```python
from build123d import *

# Parameters (mm, degrees)
SKETCH1_W                        = 99.549072562
SKETCH1_H                        = 80.386282086
EXTRUDE2_DEPTH                   = 19.05
SKETCH2_R                        = 22.2631
EXTRUDE3_DEPTH                   = 20.05
F_12_24_TAPPED_HOLE1_D           = 5.4864
F_12_24_TAPPED_HOLE1_CSINK_D     = 6.7564
F_12_24_TAPPED_HOLE1_CSINK_ANGLE = 90


with BuildPart() as part:
    # Sketch1 → Extrude2 (new body)
    with BuildSketch(Plane.XY):
        Rectangle(SKETCH1_W, SKETCH1_H)
    extrude(amount=EXTRUDE2_DEPTH)

    # Sketch2 → Extrude3 (cut, through all)
    with BuildSketch(Plane.XY.offset(19.05)):
        Circle(SKETCH2_R)
    extrude(amount=-EXTRUDE3_DEPTH, mode=Mode.SUBTRACT)

    # #12-24 Tapped Hole1 (through all)
    with Locations(Plane(origin=(49.774536281, 32.984966891, 9.857222688), x_dir=(0, 0, 1), z_dir=(1, 0, 0))):
        with Locations((0, 0), (0.189841536, 64.64104303)):
            CounterSinkHole(F_12_24_TAPPED_HOLE1_D / 2, F_12_24_TAPPED_HOLE1_CSINK_D / 2, counter_sink_angle=F_12_24_TAPPED_HOLE1_CSINK_ANGLE)


solid = part.part
```
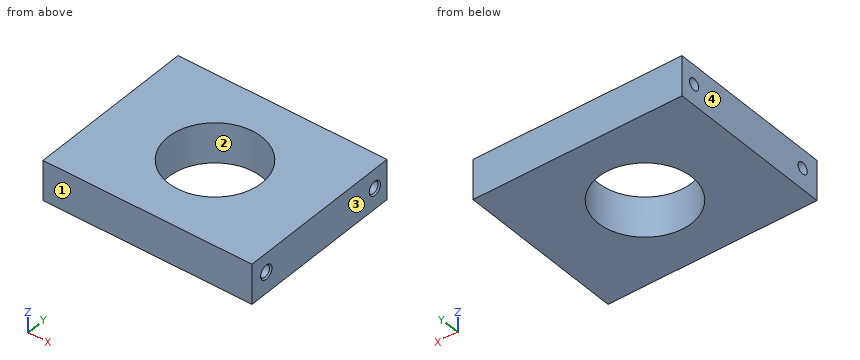
Geometry: final body of the model. Coordinates: model frame, mm. Face numbers are marked on the shaded views. Give positions to 0.01 mm unless a question says otherwise; leave off trailing zeros. Loops run counter-clockwise (first coordinate to the right, second up) from the corner with the lowest first, then second, coordinate; pieces in that order, holes last. Notation, with made-up numbers: (-22.5, 66.5) -> (-2.5, 66.5) arc R19 ccw to (-2.5, 73.5) -> close; hole circle Ø1 at (34, 37). An arc over 180 degrees is marked (long way). Return JSON: item names as keys, results as strings.
Item 1: Mould query, pull axis X, two halves, no side actions, for the marked faces 1, 2, 3 and 4. Classes: released by +X, released by -X, zero draft, split by the parting line, or undercut.
Filled in:
{"face 1": "zero draft", "face 2": "undercut", "face 3": "released by +X", "face 4": "released by -X"}
Item 2: Pin query (flat end, axial travel): P1, Ø1.5, axis at x = 20, y = 29.5, coming from the -Z side; P2, Ø5, axis at y = -31.66, z = 10.05, coming from the -X side. Return the tip coordinate at first contact, or that it passes through.
Filled in:
{"P1": "z = 0", "P2": "through"}
Item 3: Line query: line 1 (Y direction, x = -0.5, z = 17); line 2 (Y direction, x = -3, z = 11.75); line 3 (Y direction, x = 1, z = 3.75). Output: solid intervals per line, ascending.
Filled in:
{"line 1": "-40.19 to -22.26, 22.26 to 40.19", "line 2": "-40.19 to -33.81, -29.51 to -22.06, 22.06 to 31, 34.97 to 40.19", "line 3": "-40.19 to -22.24, 22.24 to 40.19"}
Item 4: Section A-A, the plane y = 0. Output: boundary loops of the cut face in (x, z), plus the area to 3 significant figures.
Filled in:
{"outline": "(-49.77, 0) -> (-22.26, 0) -> (-22.26, 19.05) -> (-49.77, 19.05) -> close; (22.26, 0) -> (49.77, 0) -> (49.77, 19.05) -> (22.26, 19.05) -> close", "area": "1,050 mm^2"}
Item 5: Section C-C, the plane z = 16.25. Output: boundary loops of the cut face in (x, y).
Filled in:
{"outline": "(-49.77, -40.19) -> (49.77, -40.19) -> (49.77, 40.19) -> (-49.77, 40.19) -> close; hole circle Ø44.53 at (0, 0)"}
Item 6: Section D-D, the plane x = 20.5. Output: boundary loops of the cut face in (y, z), plus the area to 3 significant figures.
Filled in:
{"outline": "(-40.19, 0) -> (-8.68, 0) -> (-8.68, 19.05) -> (-40.19, 19.05) -> close; (8.68, 0) -> (40.19, 0) -> (40.19, 19.05) -> (8.68, 19.05) -> close; hole circle Ø5.49 at (-31.66, 10.05); hole circle Ø5.49 at (32.98, 9.86)", "area": "1,150 mm^2"}
Item 7: Section B-B, the plane x = 8. Output: boundary loops of the cut face in (y, z), plus the area to 3 significant figures.
Filled in:
{"outline": "(-40.19, 0) -> (-20.78, 0) -> (-20.78, 19.05) -> (-40.19, 19.05) -> close; (20.78, 0) -> (40.19, 0) -> (40.19, 19.05) -> (20.78, 19.05) -> close; hole circle Ø5.49 at (-31.66, 10.05); hole circle Ø5.49 at (32.98, 9.86)", "area": "693 mm^2"}
